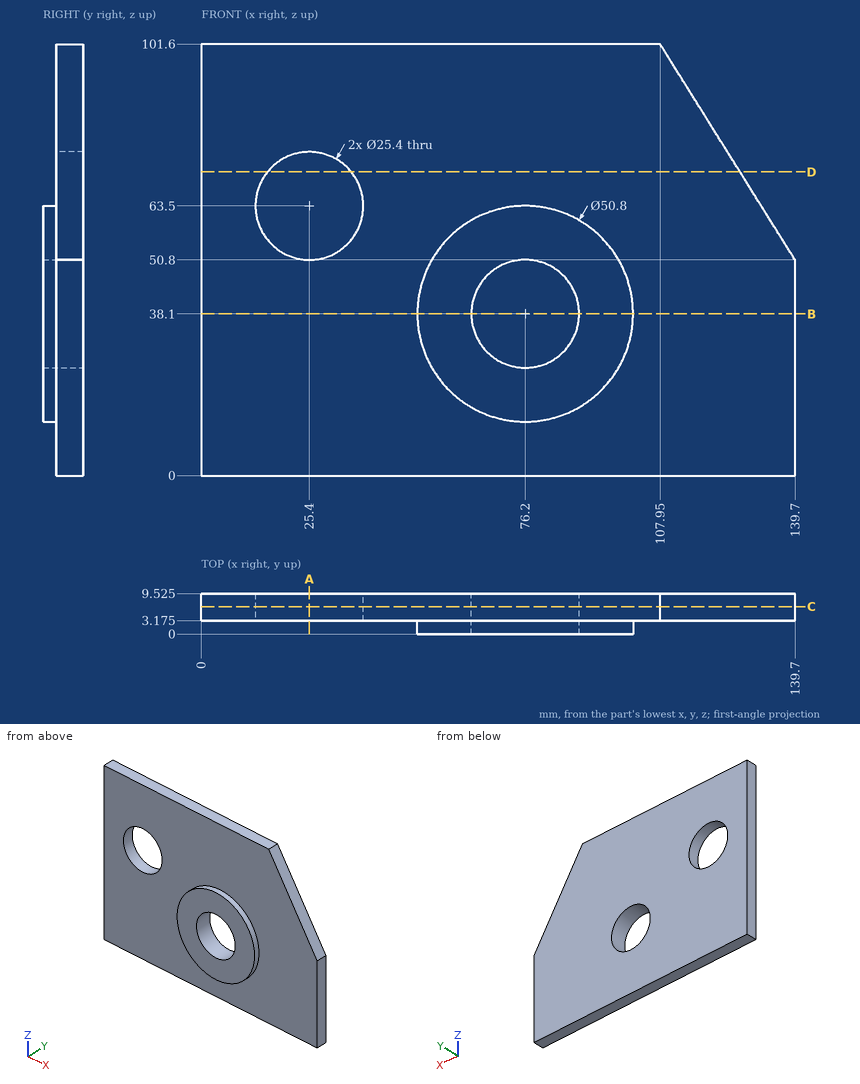
Design review of the part shown in the three views and the two pictorial views. Dimensions are in mm from the part's minimum x, y and z. Coordinates: 2 decimals unless noted, no trailing zeros. Write each loop counter-clockwise with the first axis right and the second up, starting at its lowest first coordinate (ties: lowest second). Pieces come first, ordered by that corner, then holes. Notation, with made-up numbers: (49.25, -33.75) -> (73.25, -33.75) arc R19 cw to (73.25, 1.25) -> close; hole circle Ø11 at (41, -7.75). An arc over 180 degrees is marked (long way). Answer in a Markdown table with one row per item.
1. Clearance check with flat-ended pins moving along their axes: pin 1 Ø2 at (x, z) = (42, 58.5) entering from -Y (3 decimals); pin 2 Ø1.5 at (y, z) = (7, 84) entering from +X; pin 3 Ø1.5 at (y, z) = (4.5, 76.5) entering from +X; pin 4 Ø1 at (x, z) = (60, 51.5) entering from -Y. State where each tip first meets the part, or that it passes through.
Answers below:
| item | result |
|---|---|
| pin 1 | stops at y = 3.175 |
| pin 2 | stops at x = 119.42 |
| pin 3 | stops at x = 124.11 |
| pin 4 | stops at y = 0 |
2. We need section B-B, the plane z = 38.1. State the section outline as (x, y) points (3 decimals), and give its area (3 significant figures).
Answers below:
| item | result |
|---|---|
| outline | (0, 3.175) -> (50.8, 3.175) -> (50.8, 0) -> (63.5, 0) -> (63.5, 9.525) -> (0, 9.525) -> close; (88.9, 0) -> (101.6, 0) -> (101.6, 3.175) -> (139.7, 3.175) -> (139.7, 9.525) -> (88.9, 9.525) -> close |
| area | 806 mm^2 |
3. We need section D-D, the plane z = 71.5. State the section outline as (x, y) points (1 decimal), and give its area (3 significant figures).
Answers below:
| item | result |
|---|---|
| outline | (0, 3.2) -> (15.5, 3.2) -> (15.5, 9.5) -> (0, 9.5) -> close; (35.3, 3.2) -> (126.8, 3.2) -> (126.8, 9.5) -> (35.3, 9.5) -> close |
| area | 680 mm^2 |
4. We need section C-C, the plane y = 6.5. State the section outline as (x, z) points.
Answers below:
| item | result |
|---|---|
| outline | (0, 0) -> (139.7, 0) -> (139.7, 50.8) -> (107.95, 101.6) -> (0, 101.6) -> close; hole circle Ø25.4 at (25.4, 63.5); hole circle Ø25.4 at (76.2, 38.1) |
5. We need section A-A, the plane x = 25.4. State the section outline as (y, z) points (3 decimals), and give its area (3 significant figures).
Answers below:
| item | result |
|---|---|
| outline | (3.175, 0) -> (9.525, 0) -> (9.525, 50.8) -> (3.175, 50.8) -> close; (3.175, 76.2) -> (9.525, 76.2) -> (9.525, 101.6) -> (3.175, 101.6) -> close |
| area | 484 mm^2 |
6. Wall thickness on probe 1 along Z at (x, y) = (76.2, 2.75); probe 2 along Z at (x, y) = (25.4, 7.25); probe 3 along X at (y, z) = (8.75, 40): over which ranges is each line inside the solid? List them lowest first. Write a range as [from, to].
Answers below:
| item | result |
|---|---|
| probe 1 | z = [12.7, 25.4], [50.8, 63.5] |
| probe 2 | z = [0, 50.8], [76.2, 101.6] |
| probe 3 | x = [0, 63.64], [88.76, 139.7] |
